Here's the drawing with two shaded views (mm, measured from the low corner). I have some questions. Coordinates: 2 decimals unless noted, no trailing zeros. Order: outer loops, then holes, each group sorted by start corner. A loop starts at its lowest first (then second) coordinate and runs counter-clockwise, first axis right, second up. Notation, with made-up numbers: (43.25, 85.5) -> (51.25, 85.5) arc R13 cw to (51.25, 89.5) -> close; hole circle Ø7 at (44.5, 70.5). An arc over 180 degrees is marked (long way). Answer in a Markdown table with one row per item. Add a question column.
1. Imagine slicing it at B-B on z = 21.25. Write out the boundary of the cut face in (x, y).
2. We'd pull the mould along X, two halves only. Please class the marked faces 1, 2, 3 and 4: pulls with the +X half, pulls with the -X half, needs draft (parallel to the pull), parting line crosses it, or undercut.
3. If I drill on line 1 along Z through (x, y) = (3, 5); line 2 along Y through (x, z) = (1.75, 2.5) (1 decimal); line 3 along Z through (x, y) = (6.5, 2.5), over which ranges is the centre line in solid material (lowest first)? Write a range as [from, to].
4. Imagine slicing it at A-A on x = 4. Write out the boundary of the cut face in (y, z).
5. Will these pins go through, and if not, where does the flat tip stop? pin 1 (3 mm diameter, centred on x = 4.5, z = 5, fed in from +Y); pin 2 (2 mm diameter, centred on x = 1, y = 1.5, fed in from +Z); pin 3 (3 mm diameter, centred on x = 7, z = 4, fed in from +Y); pin 4 (1.5 mm diameter, centred on x = 3.5, y = 3, fed in from -Z).
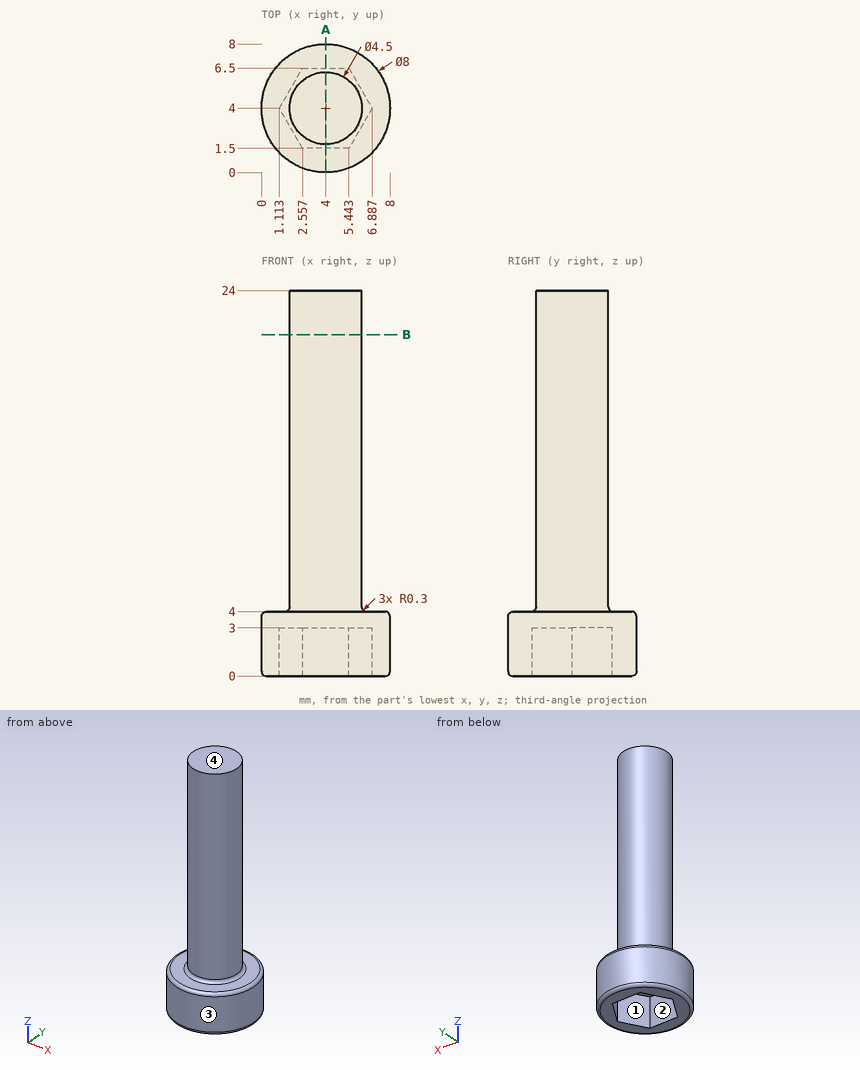
Answers follow:
| question | item | result |
|---|---|---|
| 1 | outline | circle Ø4.5 at (4, 4) |
| 2 | face 1 | undercut |
| 2 | face 2 | undercut |
| 2 | face 3 | parting line crosses it |
| 2 | face 4 | needs draft |
| 3 | line 1 | z = [3, 24] |
| 3 | line 2 | y = [0.7, 2.9], [5.1, 7.3] |
| 3 | line 3 | z = [0, 4] |
| 4 | outline | (0, 0.3) arc R0.3 ccw to (0.3, 0) -> (1.5, 0) -> (1.5, 3) -> (6.5, 3) -> (6.5, 0) -> (7.7, 0) arc R0.3 ccw to (8, 0.3) -> (8, 3.7) arc R0.3 ccw to (7.7, 4) -> (6.55, 4) arc R0.3 cw to (6.25, 4.3) -> (6.25, 24) -> (1.75, 24) -> (1.75, 4.3) arc R0.3 cw to (1.45, 4) -> (0.3, 4) arc R0.3 ccw to (0, 3.7) -> close |
| 5 | pin 1 | stops at y = 8 |
| 5 | pin 2 | stops at z = 4 |
| 5 | pin 3 | stops at y = 7.7 |
| 5 | pin 4 | stops at z = 3 |
